Check sheet for the modelled part. Datum: model origin and axes. Units: mm. Face numbers are marked on the shaded views. A direction names the side the tool comes from. Round coordinates to 2 decimals unless told otherwise and drop trailing zeros. Order: outer loops, then holes, each group sorted by start corner. A loop starts at its lowest first (then second) coordinate and runs counter-clockwise, first axis right, second up.
Q1. Scan lines: probe 1 along Y at (x, z) = (-60, -148); probe 2 along X at (y, z) = (124.5, -141.75); probe 3 along X at (y, z) = (58, -132.75). Record each from-to range of solid material in increasing order.
Q2. Set-up check for the marked faces 1 and 2: record each of +Z, -Z, +X, -X, +Y, -Y from which the full face is reachable in a straight line by a thin tool's end or side.
Q3. Cross-section at A-A on x = -60. Record the cut outline in (y, z), then the cut area to 3 significant figures.
Q4. Cross-section at D-D on z = -143.75. Record the cut outline in (x, y).
Q5. Mould release check, pull along Y, two halves, no side actions. Record for the marked faces 3, 4 and 5: +Y half, -Y half, draft (parallel to the pull), parting line (faces both ways), or undercut.
Q6. Cross-section at C-C on y = 58. Record the cut outline in (x, z), then the cut area to 4 significant figures.
Q7. Depth check by flat-ended pin: P1, Ø1, axis at x = -66.5, y = 117.5, coming from the +Z side; P2, Ø6, axis at y = 126.5, z = -131, coming from the -X side; P3, Ø2.5, axis at x = -76, y = 28.5, coming from the +Z side; P4, Ø3.5, axis at x = -70, y = 58, coming from the -Z side. Enter the tip coordinate at first touch or a pass-through.
Q8. Cross-section at B-B on z = -134. Record the cut outline in (x, y), then the cut area to 3 significant figures.
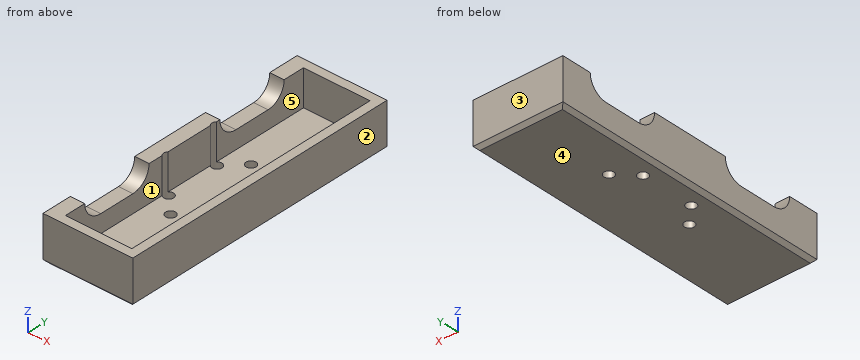
from build123d import *

# Parameters (mm, degrees)
SKETCH021_W     = 50
SKETCH021_H     = 158
PAD008_DEPTH    = 25
SKETCH022_W     = 37
SKETCH022_H     = 148
POCKET005_DEPTH = 20
POCKET006_DEPTH = 16
SKETCH024_R     = 2.75
HOLE008_DEPTH   = 25
HOLE008_TIPS_R  = 2.75
CHAMFER002_SIZE = 2


with BuildPart() as part:
    # Sketch021 → Pad008 (new body)
    with BuildSketch(Plane.XY):
        with Locations((25, 82)):
            Rectangle(SKETCH021_W, SKETCH021_H)
    extrude(amount=-PAD008_DEPTH)

    # Sketch022 → Pocket005 (cut)
    with BuildSketch(Plane.XY):
        with Locations((26.5, 82)):
            Rectangle(SKETCH022_W, SKETCH022_H)
    extrude(amount=-POCKET005_DEPTH, mode=Mode.SUBTRACT)

    # Sketch023 → Pocket006 (cut)
    with BuildSketch(Plane.YZ):
        with BuildLine():
            ThreePointArc((30.000006, 10), (20.000006, 0), (30.000006, -10))
            Line((30.000006, -10), (50, -10))
            ThreePointArc((50, -10), (60, 0), (50, 10))
            Line((30.000006, 10), (50, 10))
        make_face()
        with BuildLine():
            ThreePointArc((114.000009, 10), (104.000009, 0), (114.000009, -10))
            Line((114.000009, -10), (134, -10))
            ThreePointArc((134, -10), (144, 0), (134, 10))
            Line((114.000009, 10), (134, 10))
        make_face()
    extrude(amount=POCKET006_DEPTH, mode=Mode.SUBTRACT)

    # Sketch024 → Hole008 (cut)
    with BuildSketch(Plane.XY.offset(-25)):
        with Locations((10, 100)):
            Circle(SKETCH024_R)
        with Locations((20, 110)):
            Circle(SKETCH024_R)
        with Locations((10, 70)):
            Circle(SKETCH024_R)
        with Locations((20, 60)):
            Circle(SKETCH024_R)
    extrude(amount=HOLE008_DEPTH, mode=Mode.SUBTRACT)

    # Hole008 tips → Hole008 tip 1 section 0
    with BuildSketch(Plane.XY, mode=Mode.PRIVATE) as hole008_tip_1_s0:
        with Locations((10, 100)):
            Circle(HOLE008_TIPS_R)
    loft([hole008_tip_1_s0.sketch, Vertex(10, 100, 1.652367)], mode=Mode.SUBTRACT)

    # Hole008 tips → Hole008 tip 2 section 0
    with BuildSketch(Plane.XY, mode=Mode.PRIVATE) as hole008_tip_2_s0:
        with Locations((20, 110)):
            Circle(HOLE008_TIPS_R)
    loft([hole008_tip_2_s0.sketch, Vertex(20, 110, 1.652367)], mode=Mode.SUBTRACT)

    # Hole008 tips → Hole008 tip 3 section 0
    with BuildSketch(Plane.XY, mode=Mode.PRIVATE) as hole008_tip_3_s0:
        with Locations((10, 70)):
            Circle(HOLE008_TIPS_R)
    loft([hole008_tip_3_s0.sketch, Vertex(10, 70, 1.652367)], mode=Mode.SUBTRACT)

    # Hole008 tips → Hole008 tip 4 section 0
    with BuildSketch(Plane.XY, mode=Mode.PRIVATE) as hole008_tip_4_s0:
        with Locations((20, 60)):
            Circle(HOLE008_TIPS_R)
    loft([hole008_tip_4_s0.sketch, Vertex(20, 60, 1.652367)], mode=Mode.SUBTRACT)

    # Chamfer002
    chamfer002_edges = [part.edges().sort_by_distance(p)[0] for p in [
        (25, 3, -25),
        (0, 82, -25),
        (25, 161, -25),
        (50, 82, -25),
    ]]
    chamfer(chamfer002_edges, length=CHAMFER002_SIZE)


with BuildPart() as part_1:
    # Body006 placement: moved
    add(part.part.moved(Location((-80, -12, -126))))


solid = part_1.part
Results found:
1. probe 1: y = -9 to 45.25, 50.75 to 95.25, 100.75 to 149
1. probe 2: x = -80 to -72, -35 to -30
1. probe 3: x = -80 to -72.75, -35 to -30
2. face 1: +Z
2. face 2: +Z, -Z, +X, +Y, -Y
3. outline: (-9, -149) - (-7, -151) - (45.25, -151) - (45.25, -146) - (-4, -146) - (-4, -126) - (-9, -126) - close; (50.75, -151) - (95.25, -151) - (95.25, -146) - (50.75, -146) - close; (100.75, -151) - (147, -151) - (149, -149) - (149, -126) - (144, -126) - (144, -146) - (100.75, -146) - close
3. area: 931 mm2
4. outline: (-80, -9) - (-30, -9) - (-30, 149) - (-80, 149) - close; hole (-72, -4) - (-35, -4) - (-35, 144) - (-72, 144) - (-72, 89.89) arc R2.75 ccw to (-72, 86.11) - (-72, 59.89) arc R2.75 ccw to (-72, 56.11) - close
5. face 3: +Y half
5. face 4: draft
5. face 5: undercut
6. outline: (-80, -149) - (-78, -151) - (-72.75, -151) - (-72.75, -126) - (-80, -126) - close; (-67.25, -151) - (-32, -151) - (-30, -149) - (-30, -126) - (-35, -126) - (-35, -146) - (-67.25, -146) - close
6. area: 463.5 mm2
7. P1: stops at z = -146
7. P2: stops at x = -35
7. P3: stops at z = -136
7. P4: passes through
8. outline: (-80, -9) - (-30, -9) - (-30, 149) - (-80, 149) - (-80, 128) - (-72, 128) - (-72, 144) - (-35, 144) - (-35, -4) - (-72, -4) - (-72, 12) - (-80, 12) - close; (-80, 44) - (-72, 44) - (-72, 56.11) arc R2.75 cw to (-72, 59.89) - (-72, 86.11) arc R2.75 cw to (-72, 89.89) - (-72, 96) - (-80, 96) - close
8. area: 1,910 mm2
